Drawing for the job (mm, zero at the part's lowest x, y, z). Coordinates: 2 decimals unless noted, no trailing zeros. Loops run counter-clockwise (first coordinate to the right, second up) from the corner with the lowest first, then second, coordinate; pieces in that order, holes last. Notation, with made-up numbers: (22.5, 70.25) -> (28.5, 70.25) arc R17 cw to (28.5, 97.25) -> close; hole circle Ø3 at (6.25, -23.5). An arc over 180 degrees is marked (long way). Write each question's results on one line, items separated by ' | '.
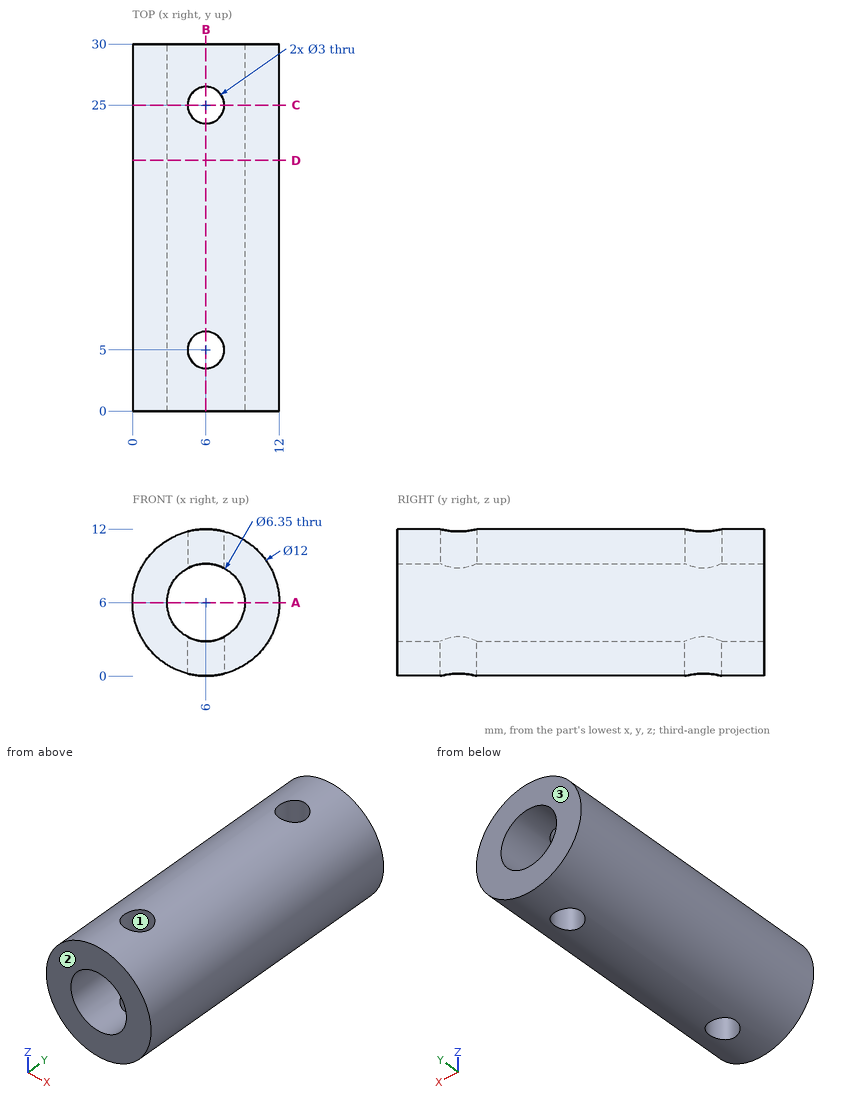
1) Slice it at A-A (z = 6). Write the cut outline in (x, y) (3 decimals).
Outcome:
outline: (0, 0) -> (2.825, 0) -> (2.825, 30) -> (0, 30) -> close; (9.175, 0) -> (12, 0) -> (12, 30) -> (9.175, 30) -> close
2) Pin check, flat tips, straight feed: pin 1 (2.5 mm diameter, centred on x = 6, y = 25, fed in from -Z); pin 2 (3 mm diameter, centred on y = 5.5, z = 1.5, fed in from -X); pin 3 (6 mm diameter, centred on x = 2.5, y = 5, fed in from +Z); pin 4 (1 mm diameter, centred on x = 8.5, y = 23, fed in from +Z). Stop position of each tip, or through.
Outcome:
pin 1: passes through | pin 2: stops at x = 0.8 | pin 3: stops at z = 11.95 | pin 4: stops at z = 11.66
3) Slice it at D-D (y = 20.5). Write the cut outline in (x, z) (3 decimals).
Outcome:
outline: circle Ø12 at (6, 6); hole circle Ø6.35 at (6, 6)
4) Slice it at C-C (y = 25). Write the cut outline in (x, z) (3 decimals), then the cut area to 3 significant figures.
Outcome:
outline: (4.5, 0.191) -> (4.5, 3.202) arc R3.175 cw to (4.5, 8.798) -> (4.5, 11.809) arc R6 ccw to start; (7.5, 0.191) arc R6 ccw to (7.5, 11.809) -> (7.5, 8.798) arc R3.175 cw to (7.5, 3.202) -> close | area: 64.1 mm^2
5) Two-plate mould, pull along Y, no slides. Class the marked faces 1, 2 and 3: pulls with the +Y half, pulls with the -Y half, needs draft (parallel to the pull), parting line crosses it, or undercut.
Outcome:
face 1: undercut | face 2: pulls with the -Y half | face 3: pulls with the +Y half
6) Slice it at B-B (x = 6). Write the cut outline in (y, z) (3 decimals).
Outcome:
outline: (0, 0) -> (3.5, 0) -> (3.5, 2.825) -> (0, 2.825) -> close; (0, 9.175) -> (3.5, 9.175) -> (3.5, 12) -> (0, 12) -> close; (6.5, 0) -> (23.5, 0) -> (23.5, 2.825) -> (6.5, 2.825) -> close; (6.5, 9.175) -> (23.5, 9.175) -> (23.5, 12) -> (6.5, 12) -> close; (26.5, 0) -> (30, 0) -> (30, 2.825) -> (26.5, 2.825) -> close; (26.5, 9.175) -> (30, 9.175) -> (30, 12) -> (26.5, 12) -> close
7) Drill centre lines: L1, parallel to Y at x = 6, z = 10.2; L2, parallel to X at y = 6, z = 5.75; L3, parallel to Z at x = 6, y = 23 (3 decimals). Where is each one in solid material? Low to high. Write a range as from..to.
Outcome:
L1: y = 0..3.5, 6.5..23.5, 26.5..30 | L2: x = 0.01..2.83, 9.17..11.99 | L3: z = 0..2.825, 9.175..12
